Autodesk Inventor part; units mm, degrees
ref_plane "Work Plane1" through (-67, 0, -11) normal (1, 0, 0) x (0, 1, 0)
ref_plane "Work Plane2" through (0, 67, -11) normal (0, 1, 0) x (-1, 0, 0)
ref_plane "XY Plane" through (0, 0, 0) normal (0, 0, 1) x (1, 0, 0)
sketch "Sketch1" plane through (0, 0, 0) normal (0, 1, 0) x (-1, 0, 0)
  line L0 (0, 0) -> (0, -51.1103) construction
  line L1 (-37.5, -17) -> (-40, -17)
  line L2 (-40, -17) -> (-40, -22)
  line L3 (-40, -22) -> (-67, -22)
  line L4 (-67, -22) -> (-67, 0)
  line L5 (-67, 0) -> (-62, 0)
  line L6 (-62, 0) -> (-62, -12)
  line L7 (-62, -12) -> (-37.5, -12)
  line L8 (-37.5, -12) -> (-37.5, -17)
  dimension "d0" = 75
  dimension "d1" = 80
  dimension "d2" = 5
  dimension "d3" = 124
  dimension "d4" = 134
  dimension "d5" = 12
  dimension "d8" = 5
revolve "Revolution1" add sketch "Sketch1" angle 360 about axis through (0, 0, 0) along (0, 0, -1)
sketch "Sketch2" plane through (0, 0, -22) normal (0, 0, -1) x (-1, 0, 0)
  line L0 (0, 0) -> (103.3512, 0)
  line L1 (0, 0) -> (37.4767, 37.4767)
  circle A0 centre (37.4767, 37.4767) radius 7.75
  circle A1 centre (0, 0) radius 44.45
  dimension "d10" = 53
  dimension "d72" = 45
  dimension "d79" = 15.5
hole "Hole1" at (-37.4767, 37.4767, -22) direction (0, 0, 1) diameter 6.647 depth 22.2 tip angle 118
pattern_circular "Circular Pattern1" count 4 over 360 about axis through (0, 0, -11) along (0, 0, 1) of "Hole1"
sketch "Sketch3" plane through (0, 0, -22) normal (0, 0, -1) x (-1, 0, 0)
  circle A0 centre (0, 0) radius 62
  line L0 (62, 0) -> (0, 0)
  line L1 (50.8134, -21.0476) -> (0, 0)
  point P0 (47.6314, 27.5)
  point P1 (0, 55)
  point P2 (-47.6314, 27.5)
  point P3 (-47.6314, -27.5)
  point P4 (0, -55)
  dimension "d25" = 55
  dimension "d37" = 22.5
hole "Hole2" at (-50.8134, -21.0476, -22) direction (0, 0, 1) diameter 7 end through all
pattern_circular "Circular Pattern2" count 8 over 360 about axis through (0, 0, -11) along (0, 0, 1) of "Hole2"
chamfer "Chamfer1" distance 1 angle 45 2 edges at (-67, 0, -22) (-67, 0, 0)
chamfer "Chamfer2" distance 0.2 angle 45 1 edges at (-40, 0, -22)
ref_plane "Work Plane1" through (-67, 0, -11) normal (1, 0, 0) x (0, 1, 0)
ref_plane "Work Plane2" through (0, 67, -11) normal (0, 1, 0) x (-1, 0, 0)
sketch "Sketch4" plane through (0, 67, -11) normal (0, 1, 0) x (-1, 0, 0)
  line L0 (66, -11) -> (-66, -11)
  point P0 (0, 11)
  point P1 (0, 4)
  point P2 (0, -11)
  dimension "d44" = 15
hole "Hole3" at (0, 67, -7) direction (0, -1, 0) diameter 4.917 end through all
sketch "Sketch5" plane through (-67, 0, -11) normal (1, 0, 0) x (0, 1, 0)
  line L0 (66, -11) -> (-66, -11)
  point P0 (0, 11)
  point P1 (0, 4)
  point P2 (0, -11)
  dimension "d52" = 15
hole "Hole4" at (-67, 0, -7) direction (1, 0, 0) diameter 4.917 end through all
sketch "Sketch6" plane through (0, 0, 0) normal (0, 0, 1) x (1, 0, 0)
  line L0 (-13.8582, 5.7403) -> (-52.1265, -86.6477)
  line L1 (-52.1265, -86.6477) -> (-24.4102, -98.1282)
  line L2 (-24.4102, -98.1282) -> (13.8582, -5.7403)
  line L3 (13.8582, -5.7403) -> (-13.8582, 5.7403)
  line L4 (0, 0) -> (26.9021, 0)
  dimension "d60" = 30
  dimension "d61" = 100
  dimension "d65" = 22.5
extrude "Extrusion1" cut sketch "Sketch6" against normal blind 16
sketch "Sketch8" plane through (0, 0, -22) normal (0, 0, -1) x (-1, 0, 0)
  circle A0 centre (-50.8134, 21.0476) radius 3.5
  circle A1 centre (-21.0476, -50.8134) radius 3.5
  circle A2 centre (50.8134, -21.0476) radius 3.5
  circle A3 centre (21.0476, 50.8134) radius 3.5
  circle A4 centre (-50.8134, 21.0476) radius 6
  circle A5 centre (21.0476, 50.8134) radius 6
  circle A6 centre (-21.0476, -50.8134) radius 6
  circle A7 centre (50.8134, -21.0476) radius 6
  point P0 (0, 0)
  dimension "d76" = 12
extrude "Extrusion3" cut sketch "Sketch8" against normal through all contours A0 | A4 | A5 | A6 | A7
properties part number "006" material "Stainless Steel, 440C"
Could you check a few things on this model? Use its own coordinates, in mm. A direction names the side the tool comes from. Give positions to 0.01 mm unless a question says otherwise; leave off trailing zeros. Order: outer loops, then holes, each group sorted by start corner. A loop starts at its lowest first (then second) coordinate and runs counter-clockwise, first axis right, second up.
Item 1: For faces 4 (the face through (-19, -46, -16)), 5 (the face through (12, -36, -17)), 6 (the face through (-0.738, -64.511, -4.655)), which set-ups out of +Z, -Z, +X, -X, +Y, -Y let a thin tool reach every point of the face, with its end or its side?
Item 2: I'm going to push flat-ended pins straight in: pin 1 (2 mm diameter, centred on x = 24, z = -6.5, fed in from +Y); pin 2 (3 mm diameter, centred on y = -48, z = -4, fed in from -X); pin 3 (12 mm diameter, centred on x = -19, y = -40, fed in from +Z). Where does each tip first touch, or does it pass through?
Item 3: I need wall thicknesses on line 1 (Z direction, x = 0, y = 63); line 2 (Y direction, x = 40.5, z = -17); line 3 (Y direction, x = 21, z = -14). Which ranges of each line are inside material? Lowest first, please.
Item 4: If we mould it in two halves opening along Y, with no side actions, what happens to faces 1 (the face through (-8.13, 36.61, -14.54)), 2 (the face through (-34.216, -43.409, -12.703)), 3 (the face through (36.019, 56.495, -10.86))? For each: pulls with the +Y half, pulls with the -Y half, needs draft (parallel to the pull), parting line crosses it, or undercut.
Item 5: If we section it at A-A, the plane z = -7: Write out the boundary of the cut face in (x, y), plus the area to 3 significant figures.
Values:
1. face 4: +Z
1. face 5: -Z
1. face 6: +Y, -Y
2. pin 1: stops at y = 62.93
2. pin 2: stops at x = -48.24
2. pin 3: stops at z = -16
3. line 1: z = -22 to -9.46, -4.54 to 0
3. line 2: y = -53.37 to -38.86, -36.1 to 36.1, 38.86 to 53.37
3. line 3: y = -63.62 to -56.81, -44.81 to -31.07, 31.07 to 47.31, 54.31 to 63.62
4. face 1: undercut
4. face 2: pulls with the -Y half
4. face 3: parting line crosses it
5. outline: (-66.95, -2.46) arc R67 ccw to (-38.85, -54.59) - (-36.88, -49.84) arc R62 cw to (-61.95, -2.46) - close; (-66.95, 2.46) - (-61.95, 2.46) arc R62 cw to (-2.46, 61.95) - (-2.46, 66.95) arc R67 ccw to start; (-11.13, -66.07) arc R67 ccw to (-2.46, -66.95) - (-2.46, -61.95) arc R62 cw to (-9.16, -61.32) - close; (2.46, -66.95) arc R67 ccw to (66.95, -2.46) - (61.95, -2.46) arc R62 cw to (2.46, -61.95) - close; (2.46, 61.95) arc R62 cw to (61.95, 2.46) - (66.95, 2.46) arc R67 ccw to (2.46, 66.95) - close
5. area: 1,780 mm2
